Part model, mm, in its own coordinate system. A direction names the side the tool comes from. Coordinates: 2 decimals unless noted, no trailing zeros. Order: outer loops, then holes, each group sorted by start corner. A loop starts at its lowest first (then second) coordinate and runs counter-clockwise, first axis right, second up. Notation, with made-up numbers: M 51,73.25 L 83,73.25 A23 cw 83,101.25 Z; hole C -6.75,12.5 d1. An arc over 180 degrees is marked long. Write item = value, one per line. Start each with the question number.
from build123d import *

# Parameters (mm, degrees)
F1_DEPTH = 32
F2_W     = 34
F2_H     = 21
F3_DEPTH = 9
F5_D     = 4.5
F5_DEPTH = 10.4
F5_TIP   = 1.3519363928


# Not quite as in the source:
# - a pattern or mirror of a feature is missing from the dataset's text; its kind, count and spacing are read off the source's solid


with BuildPart() as f1:
    # F0 (on Front) → F1 (new body, symmetric)
    with BuildSketch(Plane.XZ):
        with BuildLine():
            Line((-17, 21), (-17, 0))
            Line((-17, 0), (-7.5, 0))
            Line((-7.5, 0), (-7.5, 1.2919007565))
            ThreePointArc((-7.5, 1.2919007565), (-5, 5), (-7.5, 8.7080992435))
            Line((-7.5, 8.7080992435), (-7.5, 10))
            Line((-7.5, 10), (7.5, 10))
            Line((7.5, 10), (7.5, 8.7080992435))
            ThreePointArc((7.5, 8.7080992435), (5, 5), (7.5, 1.2919007565))
            Line((7.5, 1.2919007565), (7.5, 0))
            Line((7.5, 0), (17, 0))
            Line((17, 0), (17, 21))
            Line((17, 21), (-17, 21))
        make_face()
    extrude(amount=F1_DEPTH, both=True)

    # F2 (on face) → F3 (cut)
    with BuildSketch(Plane.XZ.offset(32)):
        with Locations((0, 10.5)):
            Rectangle(F2_W, F2_H)
        Polygon((-16.5, 19.5), (-15.5, 20.5), (15.5, 20.5), (16.5, 19.5), (16.5, 0.5), (-16.5, 0.5), align=None, mode=Mode.SUBTRACT)
    f3 = extrude(amount=-F3_DEPTH, mode=Mode.SUBTRACT)

    # F3_copies: F3 across plane
    add(f3.mirror(Plane.ZX), mode=Mode.SUBTRACT)

    # F5
    with Locations(Plane.XY.offset(21)):
        with Locations((-12.5, 12.5), (12.5, 12.5), (12.5, -12.5), (-12.5, -12.5)):
            Hole(F5_D / 2, depth=F5_DEPTH)
            with Locations((0, 0, -(F5_DEPTH + F5_TIP / 2))):  # 118° drill point
                Cone(0, F5_D / 2, F5_TIP, mode=Mode.SUBTRACT)


solid = f1.part
Item 1: Cut at B-B, the plane y = -27. Write the cut outline in (x, z).
Item 2: Flat gauge pins, fed straight in: pin 1 (4 mm diameter, centred on x = -12.5, y = -12.5, fed in from +Z); pin 2 (7 mm diameter, centred on y = -28, z = 9.5, fed in from -X); pin 3 (10 mm diameter, centred on x = -12, y = -28.5, fed in from -Z). Where does each tip first touch, or does it go through?
Item 3: Cut at C-C, the plane x = 1.5. Write the cut outline in (y, z).
Item 4: Cut at A-A, the plane z = 5.25. Write the cut outline in (x, y).
Item 5: 3-axis set-ups, long thin cutter, end or side, ignore diameter. For faces 3 (the flat face through (-12, -28, 0.5)), 4 (the flat face through (-16.5, 28, 10)), 5 (the flat face through (16.5, -28, 10)), 6 (the flat face through (0, -28, 20.5)), 7 (the flat face through (7.5, 0, 9)): which of +Z, -Z, +X, -X, +Y, -Y reach the whole face in a straight line?
Item 6: Wall check: line 1 along X through (y, z) = (-12.5, 12.5); line 2 along Y through (x, z) = (12.5, 17); line 3 along Y through (x, z) = (11.5, 14). Give the ranges that are in metal, low to high. Write a range as [from, to].
Item 7: Cut at D-D, the plane z = 18.25. Write the cut outline in (x, y).
Item 8: Pull direction Y, two halves, no side cores. Call faces 1 (the cylindrical face through (-10.84, -10.98, 15.73)), 2 (the flat face through (0, 0, 21)): pulls with the +Y half, pulls with the -Y half, needs draft (parallel to the pull), parting line crosses it, or undercut.
Filled sheet:
q1.outline = M -16.5,0.5 L -7.5,0.5 L -7.5,1.29 A4 ccw -7.5,8.71 L -7.5,10 L 7.5,10 L 7.5,8.71 A4 ccw 7.5,1.29 L 7.5,0.5 L 16.5,0.5 L 16.5,19.5 L 15.5,20.5 L -15.5,20.5 L -16.5,19.5 Z
q2.pin_1 = 10.45
q2.pin_2 = -16.5
q2.pin_3 = 0.5
q3.outline = M -32,10 L 32,10 L 32,20.5 L 23,20.5 L 23,21 L -23,21 L -23,20.5 L -32,20.5 Z
q4.outline = M -17,-23 L -16.5,-23 L -16.5,-32 L -5.01,-32 L -5.01,32 L -16.5,32 L -16.5,23 L -17,23 Z; M 5.01,-32 L 16.5,-32 L 16.5,-23 L 17,-23 L 17,23 L 16.5,23 L 16.5,32 L 5.01,32 Z
q5.face_3 = -Z, +X, -X, -Y
q5.face_4 = +Z, -Z, -X, +Y
q5.face_5 = +Z, -Z, +X, -Y
q5.face_6 = +Z, +X, -X, -Y
q5.face_7 = +Y, -Y
q6.line_1 = [-17, -14.75], [-10.25, 10.25], [14.75, 17]
q6.line_2 = [-32, -14.75], [-10.25, 10.25], [14.75, 32]
q6.line_3 = [-32, -14.52], [-10.48, 10.48], [14.52, 32]
q7.outline = M -17,-23 L -16.5,-23 L -16.5,-32 L 16.5,-32 L 16.5,-23 L 17,-23 L 17,23 L 16.5,23 L 16.5,32 L -16.5,32 L -16.5,23 L -17,23 Z; hole C -12.5,-12.5 d4.5; hole C -12.5,12.5 d4.5; hole C 12.5,-12.5 d4.5; hole C 12.5,12.5 d4.5
q8.face_1 = undercut
q8.face_2 = needs draft
